The listing builds one solid part. Answer for the finished solid, in the listing's coordinates (mm). A direction names the side the tool comes from. Coordinates: 2 decimals unless noted, no trailing zeros. Order: outer loops, then holes, each group sorted by start corner. A loop starts at its lowest first (then second) coordinate and runs counter-clockwise, first axis right, second up. Notation, with made-up numbers: (-37.5, 33.5) -> (-9.5, 33.5) arc R13 cw to (-9.5, 41.5) -> close; hole circle Ø2 at (87.25, 19.25). An arc over 180 degrees is marked (long way). Write item = value, one per line. Start each with the question number.
```python
from build123d import *

# Parameters (mm, degrees)
SKETCH1_W                  = 28.5
SKETCH1_H                  = 12
BOSS_EXTRUDE1_DEPTH        = 4.75
SKETCH2_W                  = 32.5
SKETCH2_H                  = 12
BOSS_EXTRUDE2_DEPTH        = 1.5
SKETCH3_W                  = 32.5
SKETCH3_H                  = 12
BOSS_EXTRUDE3_DEPTH        = 1.5
SKETCH4_W                  = 26.5
SKETCH4_H                  = 12
CUT_EXTRUDE1_DEPTH         = 6.25
SKETCH5_R                  = 3.5
CUTOUTS_DEPTH              = 10
SKETCH6_W                  = 20.7
SKETCH6_H                  = 35.5
SKETCH6_W_2                = 3
SKETCH6_H_2                = 32
MC_TRAY_BOSS_DEPTH         = 4.6
MC_START                   = -2.1
SKETCH7_W                  = 19
SKETCH7_H                  = 34
MC_TRAY_INTERIOR_CUT_DEPTH = 2.1
SWITCH_TRIANGLE_DEPTH      = 4.5
SWITCH_TAB_DEPTH           = 2
FILLET1_R                  = 1
CHAMFER1_SIZE              = 0.5
BOSS_EXTRUDE7_DEPTH        = 0.6


with BuildPart() as part:
    # Sketch1 → Boss-Extrude1 (new body)
    with BuildSketch(Plane.XY):
        with Locations((0, 6)):
            Rectangle(SKETCH1_W, SKETCH1_H)
    extrude(amount=-BOSS_EXTRUDE1_DEPTH)

    # Sketch2 → Boss-Extrude2 (add)
    with BuildSketch(Plane.XY):
        with Locations((0, 6)):
            Rectangle(SKETCH2_W, SKETCH2_H)
    extrude(amount=BOSS_EXTRUDE2_DEPTH)

    # Sketch3 → Boss-Extrude3 (add)
    with BuildSketch(Plane(origin=(0, 0, -4.75), x_dir=(-1, 0, 0), z_dir=(0, 0, -1))):
        with Locations((0, 6)):
            Rectangle(SKETCH3_W, SKETCH3_H)
    extrude(amount=BOSS_EXTRUDE3_DEPTH)

    # Sketch4 → Cut-Extrude1 (cut)
    with BuildSketch(Plane.XY.offset(1.5)):
        with Locations((0, 6)):
            Rectangle(SKETCH4_W, SKETCH4_H)
    extrude(amount=-CUT_EXTRUDE1_DEPTH, mode=Mode.SUBTRACT)

    # Sketch5 → Cutouts (cut)
    with BuildSketch(Plane.XY.offset(-4.75)):
        with Locations((9.25, 6)):
            Circle(SKETCH5_R)
        with BuildLine():
            Line((-9.3, 5.9), (-2.2, 5.9))
            ThreePointArc((-2.2, 5.9), (-0.5, 4.2), (-2.2, 2.5))
            Line((-2.2, 2.5), (-9.3, 2.5))
            ThreePointArc((-9.3, 2.5), (-11, 4.2), (-9.3, 5.9))
        make_face()
    extrude(amount=-CUTOUTS_DEPTH, mode=Mode.SUBTRACT)

    # Sketch6 → MC Tray Boss (add)
    with BuildSketch(Plane.XZ):
        with Locations((-5.9, -24)):
            Rectangle(SKETCH6_W, SKETCH6_H)
        with Locations((-13.9, -24.25)):
            Rectangle(SKETCH6_W_2, SKETCH6_H_2, mode=Mode.SUBTRACT)
        with Locations((2.1, -24.25)):
            Rectangle(SKETCH6_W_2, SKETCH6_H_2, mode=Mode.SUBTRACT)
    extrude(amount=-MC_TRAY_BOSS_DEPTH)

    # Sketch7 → MC Tray Interior Cut (cut)
    with BuildSketch(Plane(origin=(0, 4.6, 0), x_dir=(1, 0, 0), z_dir=(0, 1, 0)).offset(MC_START)):
        with Locations((-5.9, 23.25)):
            Rectangle(SKETCH7_W, SKETCH7_H)
    extrude(amount=MC_TRAY_INTERIOR_CUT_DEPTH, mode=Mode.SUBTRACT)

    # Sketch8 → Switch Triangle (add)
    with BuildSketch(Plane(origin=(0, 0, -6.25), x_dir=(-1, 0, 0), z_dir=(0, 0, -1))):
        Polygon((-4.45, 4.6), (-4.45, 0), (-10.554406179, 0), align=None)
    extrude(amount=SWITCH_TRIANGLE_DEPTH)

    # Sketch9 → Switch Tab (add)
    with BuildSketch(Plane(origin=(0, 0, -10.75), x_dir=(-1, 0, 0), z_dir=(0, 0, -1))):
        Polygon((-4.45, 4.6), (-6.942460212, 4.6), (-10.554406179, 1.878203487), (-10.554406179, 0), (-4.45, 0), align=None)
    extrude(amount=SWITCH_TAB_DEPTH)

    # Fillet1
    fillet1_edges = [part.edges().sort_by_distance(p)[0] for p in [
        (3.6, 1.25, -8.25),
        (0.6, 1.25, -40.25),
        (0.6, 1.25, -8.25),
        (-15.4, 1.25, -8.25),
        (-12.4, 1.25, -8.25),
        (-12.4, 1.25, -40.25),
        (16.25, 12, 0.75),
        (-16.25, 12, 0.75),
        (4.45, 2.3, -12.75),
        (16.25, 12, -5.5),
        (-16.25, 12, -5.5),
        (-13.25, 6, 1.5),
        (13.25, 6, 1.5),
        (4.45, 2.3, -41.75),
        (-16.25, 2.3, -41.75),
        (-15.4, 2.3, -40.25),
        (3.6, 2.3, -40.25),
    ]]
    fillet(fillet1_edges, radius=FILLET1_R)

    # Chamfer1
    chamfer1_edges = [part.edges().sort_by_distance(p)[0] for p in [
        (13.25, 12, -2.125),
        (13.542893219, 12, 1.207106781),
        (14.75, 12, 1.5),
        (15.957106781, 11.707106781, 1.5),
        (16.25, 5.5, 1.5),
        (-13.25, 12, -2.125),
        (-13.542893219, 12, 1.207106781),
        (-14.75, 12, 1.5),
        (-15.957106781, 11.707106781, 1.5),
        (-16.25, 5.5, 1.5),
        (-14.75, 12, 0),
        (-15.957106781, 11.707106781, 0),
        (-16.25, 5.5, 0),
        (14.75, 12, 0),
        (15.957106781, 11.707106781, 0),
        (16.25, 5.5, 0),
        (14.75, 12, -4.75),
        (15.957106781, 11.707106781, -4.75),
        (16.25, 5.5, -4.75),
        (-14.75, 12, -4.75),
        (-15.957106781, 11.707106781, -4.75),
        (-16.25, 5.5, -4.75),
        (-11, 4.2, -4.75),
        (-5.75, 2.5, -4.75),
        (-5.75, 5.9, -4.75),
        (-0.5, 4.2, -4.75),
    ]]
    chamfer(chamfer1_edges, length=CHAMFER1_SIZE)

    # Sketch10 → Boss-Extrude7 (add)
    with BuildSketch(Plane(origin=(0, 4.6, 0), x_dir=(1, 0, 0), z_dir=(0, 1, 0))):
        with BuildLine():
            Line((-12.726938069, 40.25), (-5.9, 40.25))
            Line((-5.9, 40.25), (0.926938069, 40.25))
            ThreePointArc((0.926938069, 40.25), (-5.9, 39.25), (-12.726938069, 40.25))
        make_face()
    extrude(amount=-BOSS_EXTRUDE7_DEPTH)


solid = part.part
```
Item 1: Section C-C, the plane x = -4.5 is taken. Give the vertices of the cut face in (y, z), then the cut area to 3 significant figures.
Item 2: Section D-D, the plane z = -3 is taken. Give the vertices of the cut face in (x, y), then the cut area to 4 significant figures.
Item 3: For a pull along X with two mould halves and no side action, classify faces 1 (the cylindrical face through (-15.965, 11.699, -5.757)), 2 (the flat face through (7.5, 2.3, -8.5)), 3 (the flat face through (-15.4, 2, -23)) as pulls with the +X half, pulls with the -X half, needs draft (parallel to the pull), parting line crosses it, or undercut.
Item 4: Section A-A, the plane z = -11.5 is taken. Give the vertices of the cut face in (x, y), then the cut area to 3 significant figures.
Item 5: Section B-B, the plane y = 8 is taken. Give the vertices of the cut face in (x, z), then the cut area to 3 significant figures.
Item 6: Each of these flat-tipped pins is pushed along its axis until it touches: pin 1 (1.4 mm diameter, centred on y = 3, z = -32, fed in from +X); pin 2 (0.6 mm diameter, centred on y = 1, z = -11.5, fed in from +X); pin 3 (1 mm diameter, centred on x = 5, z = -18, fed in from -Y) (3 decimals); pin 4 (2.5 mm diameter, centred on y = 5, z = -1.5, fed in from -X). Where does it stop, or does it pass through?
Item 7: Consider probe 1 along Z at (x, y) = (-14.5, 1); probe 2 along Y at (x, z) = (9, -5); probe 3 along X at (y, z) = (6, -1). Determine where each line is inside the solid, lowest interval first.
Item 8: Which of the six approach directions +Z, -Z, +X, -X, +Y, -Y give full straight-line access (tool end or side, diameter ignored) to faces 4 (the cylindrical face through (5.753, 6.154, -5.49)), 5 (the conical face through (15.733, 11.494, 0.191)), 6 (the cylindrical face through (-12.701, 1.267, -39.965))?
A:
q1.outline = (0, -41.75) -> (4.6, -41.75) -> (4.6, -39.29) -> (4, -39.29) -> (4, -40.25) -> (2.5, -40.25) -> (2.5, -5.25) -> (2, -4.75) -> (0, -4.75) -> close; (5.9, -6.25) -> (12, -6.25) -> (12, -4.75) -> (6.4, -4.75) -> (5.9, -5.25) -> close
q1.area = 105 mm^2
q2.outline = (-14.25, 0) -> (-13.25, 0) -> (-13.25, 11.5) -> (-13.75, 12) -> (-14.25, 12) -> close; (13.25, 0) -> (14.25, 0) -> (14.25, 12) -> (13.75, 12) -> (13.25, 11.5) -> close
q2.area = 23.75 mm^2
q3.face_1 = pulls with the -X half
q3.face_2 = pulls with the +X half
q3.face_3 = undercut
q4.outline = (-16.25, 0) -> (-15.4, 0) -> (-15.4, 4.6) -> (-16.25, 4.6) -> close; (-12.4, 0) -> (0.6, 0) -> (0.6, 2.5) -> (-12.4, 2.5) -> close; (3.6, 0) -> (10.55, 0) -> (10.55, 1.88) -> (6.94, 4.6) -> (3.6, 4.6) -> close
q4.area = 63.5 mm^2
q5.outline = (-16.25, -6.25) -> (6.38, -6.25) -> (6.38, -4.75) -> (-13.25, -4.75) -> (-13.25, 0.5) arc R1 ccw to (-14.25, 1.5) -> (-15.75, 1.5) -> (-16.25, 1) -> (-16.25, 0.5) -> (-15.75, 0) -> (-14.25, 0) -> (-14.25, -4.75) -> (-15.75, -4.75) -> (-16.25, -5.25) -> close; (12.12, -6.25) -> (16.25, -6.25) -> (16.25, -5.25) -> (15.75, -4.75) -> (14.25, -4.75) -> (14.25, 0) -> (15.75, 0) -> (16.25, 0.5) -> (16.25, 1) -> (15.75, 1.5) -> (14.25, 1.5) arc R1 ccw to (13.25, 0.5) -> (13.25, -4.75) -> (12.12, -4.75) -> close
q5.area = 57.5 mm^2
q6.pin_1 = 4.45
q6.pin_2 = 10.55
q6.pin_3 = through
q6.pin_4 = -14.25
q7.probe_1 = -41.75 to -40.24, -8.26 to -4.75, 0 to 1.5
q7.probe_2 = 0 to 2.51, 9.49 to 12
q7.probe_3 = -14.25 to -13.25, 13.25 to 14.25
q8.face_4 = +Z
q8.face_5 = +X, +Y
q8.face_6 = +Y, -Y
